from build123d import *

# Parameters (mm, degrees)
SKETCH1_W           = 122
SKETCH1_H           = 114
BOSS_EXTRUDE1_DEPTH = 6
SKETCH2_R           = 1.65
CUT_EXTRUDE1_DEPTH  = 6
SKETCH3_R           = 2.5
CUT_EXTRUDE2_DEPTH  = 3
SKETCH4_R           = 1.75
SKETCH4_R_2         = 2.2
CUT_EXTRUDE3_DEPTH  = 84.701851831
SKETCH5_W           = 23
SKETCH5_H           = 50
BOSS_EXTRUDE2_DEPTH = 6
SKETCH6_R           = 1.65
CUT_EXTRUDE4_DEPTH  = 124.312610872


with BuildPart() as part:
    # Sketch1 → Boss-Extrude1 (new body)
    with BuildSketch(Plane.XY):
        Rectangle(SKETCH1_W, SKETCH1_H)
    extrude(amount=BOSS_EXTRUDE1_DEPTH)

    # Sketch2 → Cut-Extrude1 (cut)
    with BuildSketch(Plane.XY.offset(6)):
        with Locations((-47.78, 53.28)):
            Circle(SKETCH2_R)
        with Locations(Location((47.78, 53.28, 0), (0, 0, 180))):
            Circle(SKETCH2_R)
        with Locations((47.78, -53.28)):
            Circle(SKETCH2_R)
        with Locations(Location((-47.78, -53.28, 0), (0, 0, 180))):
            Circle(SKETCH2_R)
    extrude(amount=-CUT_EXTRUDE1_DEPTH, mode=Mode.SUBTRACT)

    # Sketch3 → Cut-Extrude2 (cut)
    with BuildSketch(Plane.XY.offset(6)):
        with Locations((-47.78, 53.28)):
            Circle(SKETCH3_R)
        with Locations(Location((47.78, 53.28, 0), (0, 0, 180))):
            Circle(SKETCH3_R)
        with Locations((47.78, -53.28)):
            Circle(SKETCH3_R)
        with Locations(Location((-47.78, -53.28, 0), (0, 0, 180))):
            Circle(SKETCH3_R)
    extrude(amount=-CUT_EXTRUDE2_DEPTH, mode=Mode.SUBTRACT)

    # Sketch4 → Cut-Extrude3 (cut, through all)
    with BuildSketch(Plane.XY.offset(6)):
        with Locations((-53, 32)):
            Circle(SKETCH4_R)
        with Locations((-53, 17)):
            Circle(SKETCH4_R)
        with Locations((-56, -35)):
            Circle(SKETCH4_R_2)
        with Locations((-56, -45)):
            Circle(SKETCH4_R_2)
    cut_extrude3 = extrude(amount=-CUT_EXTRUDE3_DEPTH, mode=Mode.SUBTRACT)

    # Mirror1: Cut-Extrude3 across plane
    add(cut_extrude3.mirror(Plane(origin=(0, 0, 0), x_dir=(0, 0, 1), z_dir=(1, 0, 0))), mode=Mode.SUBTRACT)

    # Sketch5 → Boss-Extrude2 (add, through all)
    with BuildSketch(Plane.XY.offset(6)):
        with Locations((0, -82)):
            Rectangle(SKETCH5_W, SKETCH5_H)
    extrude(amount=-BOSS_EXTRUDE2_DEPTH)

    # Sketch6 → Cut-Extrude4 (cut, through all)
    with BuildSketch(Plane.XY.offset(6)):
        with Locations((-8, -65)):
            Circle(SKETCH6_R)
        with Locations((-8, -95)):
            Circle(SKETCH6_R)
        with Locations(Location((8, -95, 0), (0, 0, 180))):
            Circle(SKETCH6_R)
        with Locations(Location((8, -65, 0), (0, 0, 180))):
            Circle(SKETCH6_R)
    extrude(amount=-CUT_EXTRUDE4_DEPTH, mode=Mode.SUBTRACT)


solid = part.part
Check sheet for the modelled part. Datum: model origin and axes. Units: mm. A direction names the side the tool comes from. Round coordinates to 2 decimals unless told otherwise and drop trailing zeros. Order: outer loops, then holes, each group sorted by start corner. A loop starts at its lowest first (then second) coordinate and runs counter-clockwise, first axis right, second up.
(1) Cross-section at C-C, the plane z = 4.4. State how many separate pieces and enclosed holes the cut face has, and give its area (3 significant figures).
(2) Cross-section at A-A, the plane y = 53.28. Enter the section's corners in (x, z), and give its area (3 significant figures).
(3) Cross-section at B-B, the plane x = -8. Enter the section's corners in (y, z), and give its area (3 significant figures).
(4) Scan lines: probe 1 along Y at (x, z) = (47.78, 4.2); probe 2 along Y at (x, z) = (-8, 1.5); probe 3 along Y at (x, z) = (54, 3.05). Record each from-to range of solid material in increasing order.
(5) Access from +Z, -Z, +X, -X, +Y, -Y to the whole of each face (thin tool, end or side, straight path). Record for faces 4 (the flat face through (-1, 57, 3)), 5 (the cylindrical face through (-49.62, 54.97, 4.52)).
(6) Cross-section at D-D, the plane x = 47.78. Enter the section's corners in (y, z).
(7) Draft check along X on faces 1 (the flat face through (-37, -57, 3)), 2 (the flat face through (-11.5, -82, 3)), 3 (the cylindrical face through (-49.12, -55.39, 4.52)). Enter one of: pulls with the +X half, pulls with the -X half, needs draft (parallel to the pull), parting line crosses it, or undercut.
(8) Go/stop test with flat-tipped pins: P1, Ø4.5, axis at x = 47.78, y = 53.28, coming from the +Z side; P2, Ø1.8, axis at x = 40, z = 3.5, coming from the -Y side. Record where each tip stops, or that it passes through.
Check sheet entries:
1. separate pieces: 1
1. enclosed holes: 16
1. area: 14,800 mm2
2. outline: (-61, 0) - (-49.43, 0) - (-49.43, 3) - (-50.28, 3) - (-50.28, 6) - (-61, 6) - close; (-46.13, 0) - (46.13, 0) - (46.13, 3) - (45.28, 3) - (45.28, 6) - (-45.28, 6) - (-45.28, 3) - (-46.13, 3) - close; (49.43, 0) - (61, 0) - (61, 6) - (50.28, 6) - (50.28, 3) - (49.43, 3) - close
2. area: 682 mm2
3. outline: (-107, 0) - (-96.65, 0) - (-96.65, 6) - (-107, 6) - close; (-93.35, 0) - (-66.65, 0) - (-66.65, 6) - (-93.35, 6) - close; (-63.35, 0) - (57, 0) - (57, 6) - (-63.35, 6) - close
3. area: 944 mm2
4. probe 1: y = -57 to -55.78, -50.78 to 50.78, 55.78 to 57
4. probe 2: y = -107 to -96.65, -93.35 to -66.65, -63.35 to 57
4. probe 3: y = -57 to -45.92, -44.08 to -35.92, -34.08 to 15.56, 18.44 to 30.56, 33.44 to 57
5. face 4: +Z, -Z, +X, -X, +Y
5. face 5: +Z
6. outline: (-57, 0) - (-54.93, 0) - (-54.93, 3) - (-55.78, 3) - (-55.78, 6) - (-57, 6) - close; (-51.63, 0) - (51.63, 0) - (51.63, 3) - (50.78, 3) - (50.78, 6) - (-50.78, 6) - (-50.78, 3) - (-51.63, 3) - close; (54.93, 0) - (57, 0) - (57, 6) - (55.78, 6) - (55.78, 3) - (54.93, 3) - close
7. face 1: needs draft
7. face 2: pulls with the -X half
7. face 3: undercut
8. P1: stops at z = 3
8. P2: stops at y = -57
